Check sheet for the modelled part. Datum: model origin and axes. Units: mm. A direction names the side the tool comes from. Round coordinates to 2 decimals unless told otherwise and drop trailing zeros. Loops run counter-clockwise (first coordinate to the right, second up) from the corner with the lowest first, then second, coordinate; pieces in that order, holes last. Notation, with made-up numbers: (-37.75, 5) -> (-17.75, 5) arc R19 ccw to (-17.75, 16) -> close; hole circle Ø4 at (76.25, 55). An arc over 180 degrees is marked (long way). One line per item, written item: value. Start each with the question number.
1. Cross-section at D-D on x = 9. Record the cut outline in (y, z).
2. Cross-section at A-A on x = -16. Record the cut outline in (y, z).
3. Cross-section at C-C on z = 2.4. Count the separate pieces of the cut face and the enclosed holes in it, then the cut area to 3 significant figures.
4. Cross-section at B-B on y = 113. Record the cut outline in (x, z).
5. Set-up check for faces 4 (the face through (-27, -22.5, 2)), 5 (the face through (12, -12.5, 2)), 6 (the face through (-56, 103, 2)): record each of +Z, -Z, +X, -X, +Y, -Y from which the full face is reachable in a straight line by a thin tool's end or side.
6. Go/stop test with flat-tipped pins: pin 1 (2 mm diameter, centred on y = 50, z = 2.5, fed in from +X); pin 2 (3 mm diameter, centred on x = 16, y = 132, fed in from -Z); pin 3 (1.5 mm diameter, centred on x = -41, z = 3, fed in from +Y); pin 4 (1.2 mm diameter, centred on x = -13, z = 1, fed in from +Y). Record where each tip stops, or that it passes through.
7. Material ranges on L1, parallel to X at y = 113, z = 1.05; L2, parallel to Y at x = 16, z = 2.1; L3, parallel to X at y = 77.5, z = 3.35, recorded low to high.
8. Release check for a two-part mould opening along Y. For faces 1 (the face through (-40, 150, 2)), 2 (the face through (-7, 142.5, 2)), 3 (the face through (-8, 102.5, 2)) record: +Y half, -Y half, draft (parallel to the pull), parting line (faces both ways), or undercut.
from build123d import *

# Parameters (mm, degrees)
F1_DEPTH = 4
F2_D     = 5


with BuildPart() as f1:
    # F0 (on Top) → F1 (new body)
    with BuildSketch(Plane.XY):
        with BuildLine():
            ThreePointArc((0, -12.5), (-12.5, 0), (0, 12.5))
            Line((0, 12.5), (23, 12.5))
            ThreePointArc((23, 12.5), (24.4142135624, 13.0857864376), (25, 14.5))
            Line((25, 14.5), (25, 20.5))
            ThreePointArc((25, 20.5), (24.4142135624, 21.9142135624), (23, 22.5))
            Line((23, 22.5), (-35, 22.5))
            ThreePointArc((-35, 22.5), (-38.5355339059, 23.9644660941), (-40, 27.5))
            Line((-40, 27.5), (-40, 97.5))
            ThreePointArc((-40, 97.5), (-38.5355339059, 101.0355339059), (-35, 102.5))
            Line((-35, 102.5), (20, 102.5))
            ThreePointArc((20, 102.5), (23.5355339059, 103.9644660941), (25, 107.5))
            Line((25, 107.5), (25, 137.5))
            ThreePointArc((25, 137.5), (23.5355339059, 141.0355339059), (20, 142.5))
            Line((20, 142.5), (-35, 142.5))
            ThreePointArc((-35, 142.5), (-38.5355339059, 143.9644660941), (-40, 147.5))
            Line((-40, 147.5), (-40, 152.5))
            ThreePointArc((-40, 152.5), (-41.4644660941, 156.0355339059), (-45, 157.5))
            Line((-45, 157.5), (-75, 157.5))
            ThreePointArc((-75, 157.5), (-78.5355339059, 156.0355339059), (-80, 152.5))
            Line((-80, 152.5), (-80, -17.5))
            ThreePointArc((-80, -17.5), (-78.5355339059, -21.0355339059), (-75, -22.5))
            Line((-75, -22.5), (23, -22.5))
            ThreePointArc((23, -22.5), (24.4142135624, -21.9142135624), (25, -20.5))
            Line((25, -20.5), (25, -14.5))
            ThreePointArc((25, -14.5), (24.4142135624, -13.0857864376), (23, -12.5))
            Line((23, -12.5), (0, -12.5))
        make_face()
        with BuildLine():
            Line((-64, 57.5), (-64, 147.5))
            ThreePointArc((-64, 147.5), (-60, 151.5), (-56, 147.5))
            Line((-56, 147.5), (-56, 57.5))
            ThreePointArc((-56, 57.5), (-60, 53.5), (-64, 57.5))
        make_face(mode=Mode.SUBTRACT)
    extrude(amount=F1_DEPTH)

    # F2 (through all)
    with Locations(Plane(origin=(0, 0, 0), x_dir=(1, 0, 0), z_dir=(0, 0, -1))):
        with Locations((-16, -132), (16, -132), (16, -113), (-16, -113)):
            Hole(F2_D / 2)


solid = f1.part
Taken from the geometry:
1. outline: (-22.5, 0) -> (-12.5, 0) -> (-12.5, 4) -> (-22.5, 4) -> close; (12.5, 0) -> (22.5, 0) -> (22.5, 4) -> (12.5, 4) -> close; (102.5, 0) -> (142.5, 0) -> (142.5, 4) -> (102.5, 4) -> close
2. outline: (-22.5, 0) -> (22.5, 0) -> (22.5, 4) -> (-22.5, 4) -> close; (102.5, 0) -> (110.5, 0) -> (110.5, 4) -> (102.5, 4) -> close; (115.5, 0) -> (129.5, 0) -> (129.5, 4) -> (115.5, 4) -> close; (134.5, 0) -> (142.5, 0) -> (142.5, 4) -> (134.5, 4) -> close
3. separate pieces: 1
3. enclosed holes: 5
3. area: 11,000 mm2
4. outline: (-80, 0) -> (-64, 0) -> (-64, 4) -> (-80, 4) -> close; (-56, 0) -> (-18.5, 0) -> (-18.5, 4) -> (-56, 4) -> close; (-13.5, 0) -> (13.5, 0) -> (13.5, 4) -> (-13.5, 4) -> close; (18.5, 0) -> (25, 0) -> (25, 4) -> (18.5, 4) -> close
5. face 4: +Z, -Z, +X, -X, -Y
5. face 5: +Z, -Z, +X
5. face 6: +Z, -Z
6. pin 1: stops at x = -40
6. pin 2: passes through
6. pin 3: stops at y = 156.3
6. pin 4: stops at y = 142.5
7. L1: x = -80 to -64, -56 to -18.5, -13.5 to 13.5, 18.5 to 25
7. L2: y = -22.5 to -12.5, 12.5 to 22.5, 102.5 to 110.5, 115.5 to 129.5, 134.5 to 142.5
7. L3: x = -80 to -64, -56 to -40
8. face 1: draft
8. face 2: +Y half
8. face 3: undercut
